Check sheet for the modelled part. Datum: model origin and axes. Units: mm. Face numbers are marked on the shaded views. A direction names the side the tool comes from. Coordinates: 2 decimals unless noted, no trailing zeros. Loops run counter-clockwise (first coordinate to the right, second up) from the corner with the lowest first, then second, coordinate; pieces in that order, holes last. Notation, with made-up numbers: M 86.5,48.5 L 114.5,48.5 A22 cw 114.5,65.5 Z; hole C -7.5,-30.75 d6. An arc over 180 degrees is marked long. Return JSON: item names as keys, results as strings.
from build123d import *

# Parameters (mm, degrees)
F0_W     = 122.128874
F0_H     = 74.222378
F1_DEPTH = 71.6
F2_T     = -2.5
F3_W     = 117.128874
F3_H     = 69.1
F4_DEPTH = 25


with BuildPart() as f1:
    # F0 (on Top) → F1 (new body)
    with BuildSketch(Plane.XY):
        with Locations((61.064437, 37.111189)):
            Rectangle(F0_W, F0_H)
    extrude(amount=F1_DEPTH)

    # F2
    f2_openings = [f1.faces().sort_by_distance(p)[0] for p in [
        (61.064437, 37.111189, 71.6),
    ]]
    offset(amount=F2_T, openings=f2_openings)

    # F3 (on face) → F4 (cut)
    with BuildSketch(Plane(origin=(0, 74.222378, 0), x_dir=(-1, 0, 0), z_dir=(0, 1, 0))):
        with Locations((-61.064437, 37.05)):
            Rectangle(F3_W, F3_H)
    extrude(amount=-F4_DEPTH, mode=Mode.SUBTRACT)


solid = f1.part
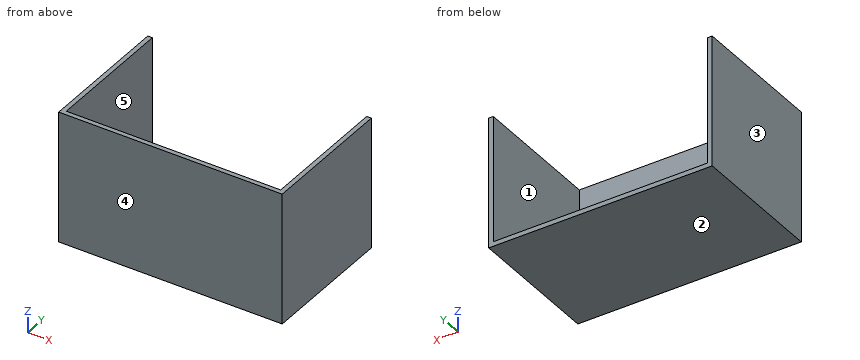
1) Section check B-B on x = 61.5. Record the cut outline in (y, z), then the cut area to 3 significant figures.
Answers:
{"outline": "M 0,0 L 74.22,0 L 74.22,2.5 L 2.5,2.5 L 2.5,71.6 L 0,71.6 Z", "area": "358 mm²"}
2) Section check A-A on y = 57.5. Record the cut outline in (x, z), then the cut area to 3 significant figures.
Answers:
{"outline": "M 0,0 L 122.13,0 L 122.13,71.6 L 119.63,71.6 L 119.63,2.5 L 2.5,2.5 L 2.5,71.6 L 0,71.6 Z", "area": "651 mm²"}
3) Draft check along X on the marked faces 1, 2 and 3. Enter one of: +X half, -X half, draft (parallel to the pull), parting line (faces both ways), or undercut.
Answers:
{"face 1": "undercut", "face 2": "draft", "face 3": "-X half"}
4) Section check C-C on z = 25. Record the cut outline in (x, y).
Answers:
{"outline": "M 0,0 L 122.13,0 L 122.13,74.22 L 119.63,74.22 L 119.63,2.5 L 2.5,2.5 L 2.5,74.22 L 0,74.22 Z"}
5) Set-up check for the marked faces 4 and 5: record each of +Z, -Z, +X, -X, +Y, -Y from which the full face is reachable in a straight line by a thin tool's end or side.
Answers:
{"face 4": "+Z, -Z, +X, -X, -Y", "face 5": "+Z, +Y"}
6) Scan lines: line 1 along X through (y, z) = (54, 39); line 2 along Y through (x, z) = (116, 38). Record each from-to range of solid material in increasing order. Write a range as [from, to].
Answers:
{"line 1": "[0, 2.5], [119.63, 122.13]", "line 2": "[0, 2.5]"}
7) Go/stop test with flat-tipped pins: pin 1 Ø8 at (x, z) = (64.5, 46.5) entering from +Y; pin 2 Ø5 at (x, y) = (84, 62) entering from +Z. Record where each tip stops, or that it passes through.
Answers:
{"pin 1": "y = 2.5", "pin 2": "z = 2.5"}
